Design review of the part shown in the three views and the two pictorial views. Dimensions are in mm from the part's minimum x, y and z. Round coordinates to 2 decimals unless told otherwise and drop trailing zeros. Loops run counter-clockwise (first coordinate to the right, second up) from the corner with the lowest first, then second, coordinate; pieces in that order, holes last.
1) Wall thickness on L1, parallel to X at y = 1.5, z = 25; L2, parallel to Z at x = 31, y = 2.1; L3, parallel to X at y = 2.6, z = 21.75: over which ranges is each line inside the solid? List them lowest first.
2) Take a section at A-A (z = 25). State the section outline as (x, y) points.
3) Take a section at C-C (y = 1.1). State the section outline as (x, z) points, then the cut area to 3 significant figures.
4) Take a section at B-B (x = 81). State the section outline as (y, z) points.
5) Insertion check: pin 1 (1.5 mm diameter, centred on y = 3.5, z = 18, fed in from +X); pin 2 (2.5 mm diameter, centred on x = 81, z = 25, fed in from -Y). Each pin has a flat end and moves straight along its axis. Give the tip position at first contact, or say it passes through.
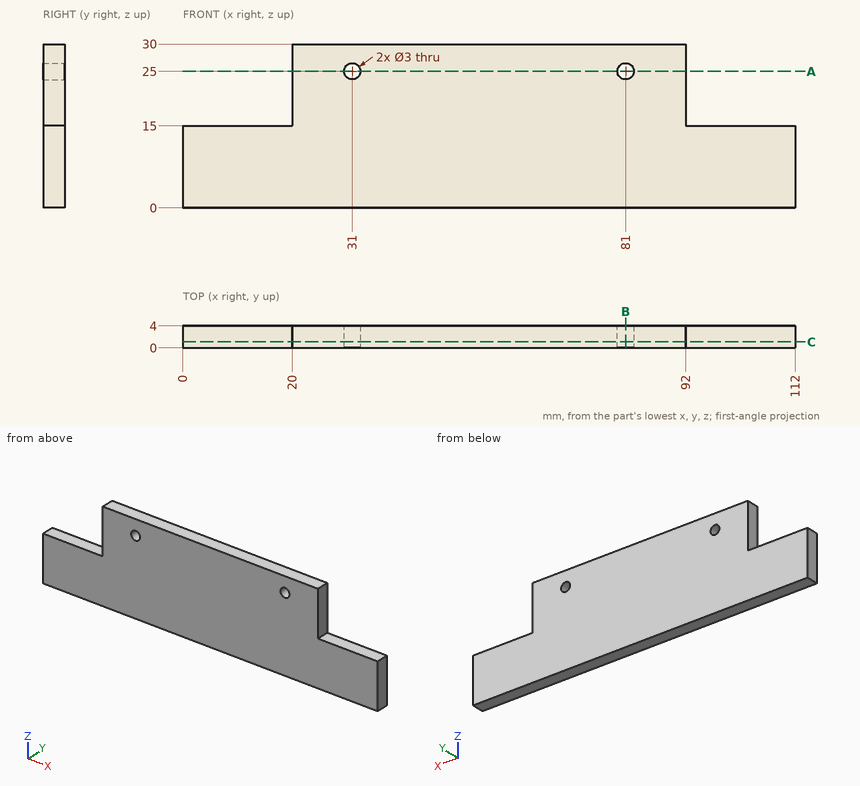
Response:
1. L1: x = 20 to 29.5, 32.5 to 79.5, 82.5 to 92
1. L2: z = 0 to 23.5, 26.5 to 30
1. L3: x = 20 to 92
2. outline: (20, 0) - (29.5, 0) - (29.5, 4) - (20, 4) - close; (32.5, 0) - (79.5, 0) - (79.5, 4) - (32.5, 4) - close; (82.5, 0) - (92, 0) - (92, 4) - (82.5, 4) - close
3. outline: (0, 0) - (112, 0) - (112, 15) - (92, 15) - (92, 30) - (20, 30) - (20, 15) - (0, 15) - close; hole circle Ø3 at (31, 25); hole circle Ø3 at (81, 25)
3. area: 2,750 mm2
4. outline: (0, 0) - (4, 0) - (4, 23.5) - (0, 23.5) - close; (0, 26.5) - (4, 26.5) - (4, 30) - (0, 30) - close
5. pin 1: stops at x = 92
5. pin 2: passes through
